Work out the finished part from the listing and answer in its coordinate system (mm). A direction names the side the tool comes from. Round coordinates to 2 decimals unless told otherwise and drop trailing zeros. Write each loop counter-clockwise with the first axis right and the second up, starting at its lowest first coordinate (ties: lowest second). Pieces come first, ordered by that corner, then holes.
1. Find section A-A (z = 0.75). Write down the section's boundary in (x, y).
2. Find section B-B (z = -3.75). Write down the section's boundary in (x, y), and give its area (3 significant figures).
3. A tool of negligible diameter and unlimited length cuts with its end or side. For faces 4 (the face through (-2.163, -102.518, 2.215)), 5 (the face through (-9.02, -54.39, -4.96)), 6 (the face through (-6.053, -61.455, 0.021)), from which of +Z, -Z, +X, -X, +Y, -Y can it reach the whole face along a straight path? Write none if from no direction.
4. Flat-ended cylindrical pins translate along their axes: pin 1 Ø1 at (x, z) = (-0.5, -0.5) entering from +Y; pin 2 Ø19.5 at (x, y) = (6, -96) entering from -Z; pin 3 Ø1.5 at (y, z) = (-99, -2) entering from -X. Find the tip coordinate at first contact, or state that the pin passes through.
5. Determine the mould class of faces 1 (the face through (-12, -52, -7.5)), 2 (the face through (-14.42, -45.94, 0.02)), 3 (the face through (-11, -51, -2.5)) for opening direction X: pulls with the +X half, pulls with the -X half, needs draft (parallel to the pull), parting line crosses it, or undercut.
6. Straight lines are drawn through the part: probe 1 along Y at (x, z) = (-10, -3.95); probe 2 along Y at (x, z) = (-10, -6.7); probe 3 along Z at (x, y) = (2, -92). For each, find the intervals that lie inside material, in ascending order.
```python
from build123d import *

# Parameters (mm, degrees)
SKETCH2_R           = 2
BOSS_EXTRUDE1_DEPTH = 2.5
FILLET1_R           = 1
SKETCH3_R           = 4.5
BOSS_EXTRUDE2_DEPTH = 5
SKETCH4_R           = 2.5
CUT_EXTRUDE1_DEPTH  = 3
SKETCH5_R           = 1
CUT_EXTRUDE2_DEPTH  = 5


with BuildPart() as part:
    # Sketch2 → Boss-Extrude1 (new body, symmetric)
    with BuildSketch(Plane.XY):
        with BuildLine():
            Line((-10, -126), (-5, -127.601468854))
            Line((-5, -127.601468854), (23.717421377, -82.972253802))
            ThreePointArc((23.717421377, -82.972253802), (25.211420403, -76.174808821), (21.908456188, -70.048821656))
            Line((21.908456188, -70.048821656), (-6.039708144, -45.492662824))
            ThreePointArc((-6.039708144, -45.492662824), (-14.507337176, -46.039708144), (-13.960291856, -54.507337176))
            Line((-13.960291856, -54.507337176), (2.078857085, -68.599850882))
            ThreePointArc((2.078857085, -68.599850882), (5.116155087, -73.445037833), (5.001799686, -79.162374502))
            Line((5.001799686, -79.162374502), (-10, -126))
        make_face()
        with Locations((-10, -50)):
            Circle(SKETCH2_R, mode=Mode.SUBTRACT)
    extrude(amount=BOSS_EXTRUDE1_DEPTH, both=True)

    # Fillet1
    fillet1_edges = [part.edges().sort_by_distance(p)[0] for p in [
        (25.211420403, -76.174808821, -2.5),
        (9.358710688, -105.286861328, -2.5),
        (-7.5, -126.800734427, -2.5),
        (-2.499100157, -102.581187251, -2.5),
        (9.358710688, -105.286861328, 2.5),
        (-5, -127.601468854, 0),
        (-10, -126, 0),
        (25.211420403, -76.174808821, 2.5),
        (7.934374022, -57.77074224, 2.5),
        (-14.507337176, -46.039708144, 2.5),
        (-5.940717386, -61.553594029, 2.5),
        (5.116155087, -73.445037833, 2.5),
        (-2.499100157, -102.581187251, 2.5),
        (5.116155087, -73.445037833, -2.5),
        (-7.5, -126.800734427, 2.5),
        (-5.940717386, -61.553594029, -2.5),
        (-14.507337176, -46.039708144, -2.5),
        (7.934374022, -57.77074224, -2.5),
    ]]
    fillet(fillet1_edges, radius=FILLET1_R)

    # Sketch3 → Boss-Extrude2 (add)
    with BuildSketch(Plane(origin=(0, 0, -2.5), x_dir=(-1, 0, 0), z_dir=(0, 0, -1))):
        with Locations((10, -50)):
            Circle(SKETCH3_R)
    extrude(amount=BOSS_EXTRUDE2_DEPTH)

    # Sketch4 → Cut-Extrude1 (cut)
    with BuildSketch(Plane(origin=(0, 0, -7.5), x_dir=(-1, 0, 0), z_dir=(0, 0, -1))):
        with Locations((10, -50)):
            Circle(SKETCH4_R)
    extrude(amount=-CUT_EXTRUDE1_DEPTH, mode=Mode.SUBTRACT)

    # Sketch5 → Cut-Extrude2 (cut)
    with BuildSketch(Plane.XY.offset(-2.5)):
        with Locations((-10, -50)):
            Circle(SKETCH5_R)
    extrude(amount=-CUT_EXTRUDE2_DEPTH, mode=Mode.SUBTRACT)


solid = part.part
```
Worked answers:
1. outline: (-13.96, -54.51) - (2.08, -68.6) arc R10 cw to (5, -79.16) - (-9.69, -125.05) arc R1 ccw to (-9.05, -126.31) - (-5.73, -127.37) arc R1 ccw to (-4.58, -126.96) - (23.72, -82.97) arc R10 ccw to (21.91, -70.05) - (-6.04, -45.49) arc R6 ccw to start; hole circle Ø4 at (-10, -50)
2. outline: circle Ø9 at (-10, -50); hole circle Ø2 at (-10, -50)
2. area: 60.5 mm2
3. face 4: +Z, -X
3. face 5: -Z
3. face 6: +Z, -Z, -X
4. pin 1: stops at y = -49.92
4. pin 2: stops at z = -2.5
4. pin 3: stops at x = -1.55
5. face 1: needs draft
5. face 2: parting line crosses it
5. face 3: undercut
6. probe 1: y = -54.5 to -51, -49 to -45.5
6. probe 2: y = -54.5 to -52.5, -47.5 to -45.5
6. probe 3: z = -2.5 to 2.5
